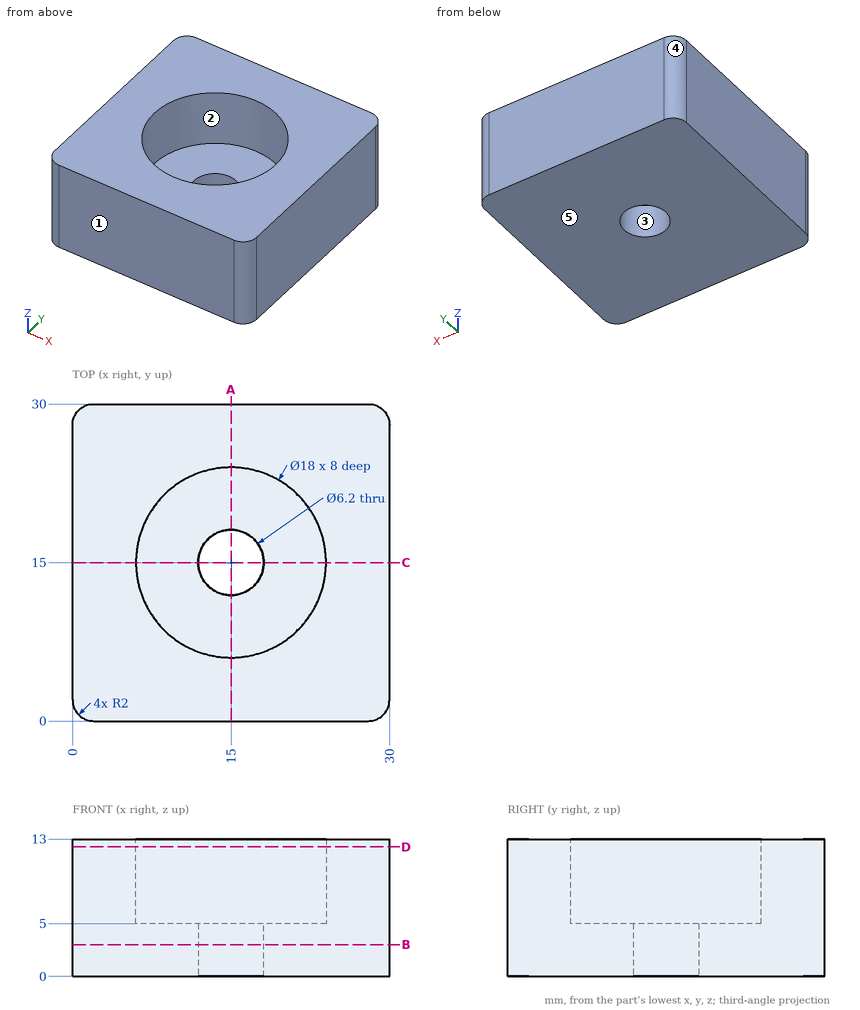
Design review of the part shown in the three views and the two pictorial views. Dimensions are in mm from the part's minimum x, y and z. A direction names the side the tool comes from. Give positions to 0.01 mm unless a question says otherwise; leave off trailing zeros. Order: outer loops, then holes, each group sorted by start corner. A loop starts at its lowest first (then second) coordinate and runs counter-clockwise, first axis right, second up. Notation, with made-up numbers: M 38,-22 L 77,-22 A32 cw 77,12 Z; hole C -8.5,44 d7. An arc over 180 degrees is marked long. Answer in a Markdown table with one row per item. Add a question column.
(1) Consider section B-B on z = 3. State the section outline as (x, y) points, and give its area (3 significant figures).
(2) Consider section A-A on x = 15. State the section outline as (y, z) points, and give its area (3 significant figures).
(3) Mouldability with a two-part tool opening along Y and no side actions: class the marked faces 3, 4 and 5 as +Y half, -Y half, draft (parallel to the pull), parting line (faces both ways), or undercut.
(4) For the marked faces 1 and 2, list the 3-axis set-ups (+Z, -Z, +X, -X, +Y, -Y) from which the entire face can be reached by the end or side of a thin tool; tool diameter is ignored.
(5) Wall thickness on probe 1 along X at (y, z) = (15, 1.35); probe 2 along Y at (x, z) = (15, 10.5): over which ranges is each line inside the solid? List them lowest first. Write a range as [from, to].
(6) Consider section D-D on z = 12.25. State the section outline as (x, y) points, and give its area (3 significant figures).
(7) For pin 1 (16 mm diameter, centred on x = 15, y = 15, fed in from +Z); pin 2 (5 mm diameter, centred on x = 15, y = 15, fed in from +Z), all flat-tipped, find the tip position at first contact; note any pin that passes through.
Evaluation:
| question | item | result |
|---|---|---|
| 1 | outline | M 0,2 A2 ccw 2,0 L 28,0 A2 ccw 30,2 L 30,28 A2 ccw 28,30 L 2,30 A2 ccw 0,28 Z; hole C 15,15 d6.2 |
| 1 | area | 866 mm^2 |
| 2 | outline | M 0,0 L 11.9,0 L 11.9,5 L 6,5 L 6,13 L 0,13 Z; M 18.1,0 L 30,0 L 30,13 L 24,13 L 24,5 L 18.1,5 Z |
| 2 | area | 215 mm^2 |
| 3 | face 3 | undercut |
| 3 | face 4 | +Y half |
| 3 | face 5 | draft |
| 4 | face 1 | +Z, -Z, +X, -X, -Y |
| 4 | face 2 | +Z |
| 5 | probe 1 | x = [0, 11.9], [18.1, 30] |
| 5 | probe 2 | y = [0, 6], [24, 30] |
| 6 | outline | M 0,2 A2 ccw 2,0 L 28,0 A2 ccw 30,2 L 30,28 A2 ccw 28,30 L 2,30 A2 ccw 0,28 Z; hole C 15,15 d18 |
| 6 | area | 642 mm^2 |
| 7 | pin 1 | stops at z = 5 |
| 7 | pin 2 | passes through |
